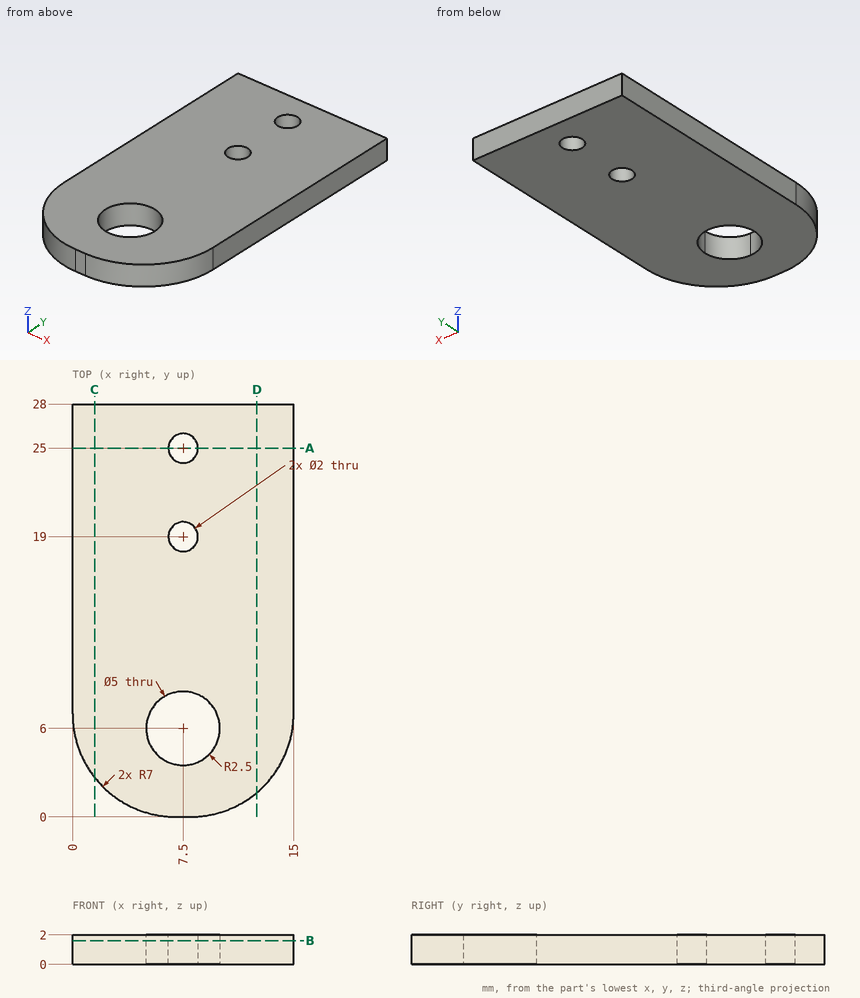
Could you check a few things on this drawing? It's one solid part, dimensions in mm from its lowest x, y, z. Round coordinates to 2 decimals unless told otherwise and drop trailing zeros. Order: outer loops, then holes, each group sorted by start corner. A loop starts at its lowest first (then second) coordinate and runs counter-clockwise, first axis right, second up. Notation, with made-up numbers: M 13.5,55.5 L 25.5,55.5 A5 ccw 25.5,61.5 Z; hole C 15,21.25 d6. An arc over 180 degrees is marked long. One line per item, written item: value.
(1) Imagine slicing it at B-B (z = 1.6). Write out the boundary of the cut face in (x, y).
Ans:
outline: M 0,7 A7 ccw 7,0 L 8,0 A7 ccw 15,7 L 15,28 L 0,28 Z; hole C 7.5,6 d5; hole C 7.5,19 d2; hole C 7.5,25 d2
(2) Imagine slicing it at C-C (x = 1.5). Write out the boundary of the cut face in (y, z), and give its area (3 significant figures).
Ans:
outline: M 2.67,0 L 28,0 L 28,2 L 2.67,2 Z
area: 50.7 mm^2
(3) I'm going to push flat-ended pins straight in: P1, Ø1.5, axis at x = 6.5, y = 4.5, coming from the -Z side; P2, Ø1, axis at x = 9.5, z = 0.5, coming from the -Y side; P3, Ø4.5, axis at x = 7.5, y = 6, coming from the -Z side. Where does each tip first touch, or does it pass through?
Ans:
P1: stops at z = 0
P2: stops at y = 0.07
P3: passes through
(4) Imagine slicing it at A-A (y = 25). Write out the boundary of the cut face in (x, z), and give its area (3 significant figures).
Ans:
outline: M 0,0 L 6.5,0 L 6.5,2 L 0,2 Z; M 8.5,0 L 15,0 L 15,2 L 8.5,2 Z
area: 26.0 mm^2
(5) I need wall thicknesses on line 1 along Y through (x, z) = (7, 1.75); line 2 along Y through (x, z) = (5.5, 1.6); line 3 along X through (y, z) = (7.25, 1.65). Which ranges of each line are inside material? Lowest first, please. Write a range as from..to.
Ans:
line 1: y = 0..3.55, 8.45..18.13, 19.87..24.13, 25.87..28
line 2: y = 0.16..4.5, 7.5..28
line 3: x = 0..5.33, 9.67..15
(6) Imagine slicing it at D-D (x = 12.5). Write out the boundary of the cut face in (y, z), and give its area (3 significant figures).
Ans:
outline: M 1.64,0 L 28,0 L 28,2 L 1.64,2 Z
area: 52.7 mm^2
